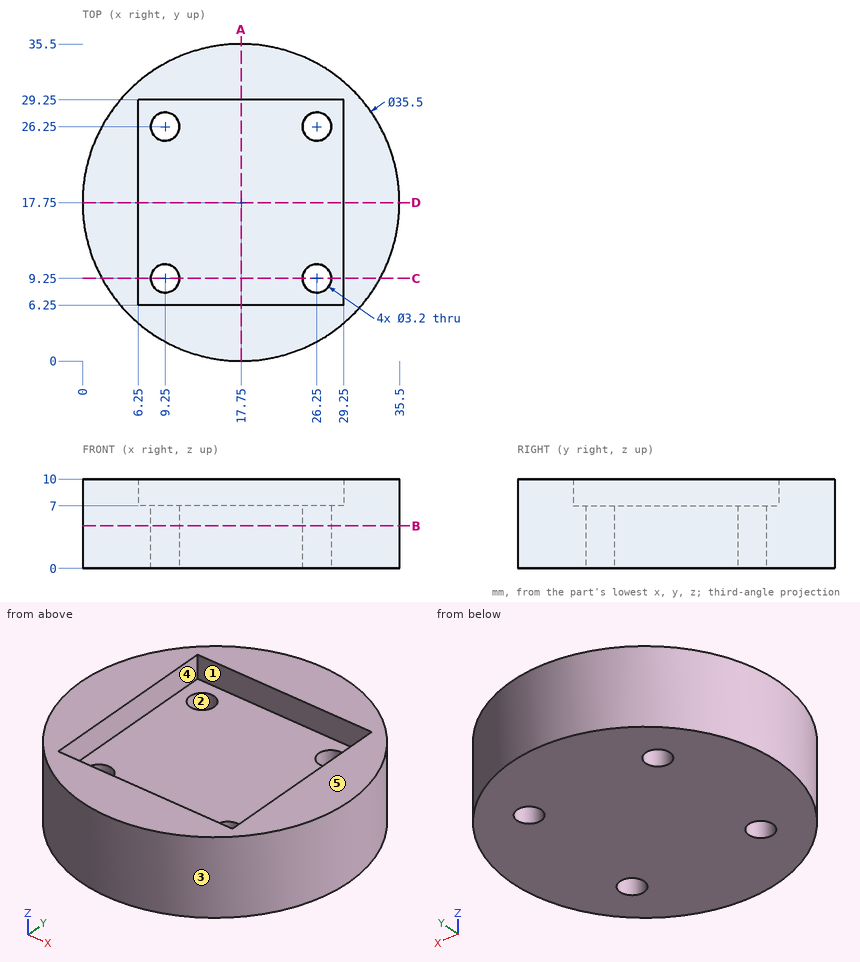
Here's the drawing with two shaded views (mm, measured from the low corner). I have some questions. A direction names the side the tool comes from. Give positions to 0.01 mm unless a question says otherwise; leave off trailing zeros. Order: outer loops, then holes, each group sorted by start corner. A loop starts at its lowest first (then second) coordinate and runs counter-clockwise, first axis right, second up. Notation, with made-up numbers: (-17, 2.25) -> (-4, 2.25) arc R32 cw to (-4, 35.25) -> close; hole circle Ø1 at (40, 17). An arc over 180 degrees is marked (long way). Use a Markdown table: item, result. Add a question column.
Item 1: I need wall thicknesses on line 1 (Y direction, x = 9.25, z = 5.25); line 2 (Y direction, x = 18, z = 8.25). Which ranges of each line are inside material? Lowest first, please.
Item 2: Will these pins go through, and if not, where does the flat tip stop? pin 1 (2.5 mm diameter, centred on x = 20, z = 8, fed in from +Y); pin 2 (2 mm diameter, centred on x = 25.5, z = 5.5, fed in from -Y); pin 3 (1.5 mm diameter, centred on y = 21.5, z = 9, fed in from +X).
Item 3: For the marked faces 1 and 2, which set-ups out of +Z, -Z, +X, -X, +Y, -Y let a thin tool reach every point of the face, with its end or its side?
Item 4: Imagine slicing it at A-A on x = 17.75. Please give me the cut outline in (y, z).
Item 5: Imagine slicing it at B-B on z = 4.75. Please give me the cut outline in (x, y), plus the area to 3 significant figures.
Item 6: Imagine slicing it at C-C on y = 9.25. Please give me the cut outline in (x, z).
Item 7: If we mould it in two halves opening along X, with no side actions, what happens to the marked faces 3, 4 and 5? For each: pulls with the +X half, pulls with the -X half, needs draft (parallel to the pull), parting line crosses it, or undercut.
Data:
| question | item | result |
|---|---|---|
| 1 | line 1 | y = 2.17 to 7.65, 10.85 to 24.65, 27.85 to 33.33 |
| 1 | line 2 | y = 0 to 6.25, 29.25 to 35.5 |
| 2 | pin 1 | stops at y = 35.47 |
| 2 | pin 2 | stops at y = 1.33 |
| 2 | pin 3 | stops at x = 35.24 |
| 3 | face 1 | +Z |
| 3 | face 2 | +Z, -Z |
| 4 | outline | (0, 0) -> (35.5, 0) -> (35.5, 10) -> (29.25, 10) -> (29.25, 7) -> (6.25, 7) -> (6.25, 10) -> (0, 10) -> close |
| 5 | outline | circle Ø35.5 at (17.75, 17.75); hole circle Ø3.2 at (9.25, 9.25); hole circle Ø3.2 at (9.25, 26.25); hole circle Ø3.2 at (26.25, 9.25); hole circle Ø3.2 at (26.25, 26.25) |
| 5 | area | 958 mm² |
| 6 | outline | (2.17, 0) -> (7.65, 0) -> (7.65, 7) -> (6.25, 7) -> (6.25, 10) -> (2.17, 10) -> close; (10.85, 0) -> (24.65, 0) -> (24.65, 7) -> (10.85, 7) -> close; (27.85, 0) -> (33.33, 0) -> (33.33, 10) -> (29.25, 10) -> (29.25, 7) -> (27.85, 7) -> close |
| 7 | face 3 | parting line crosses it |
| 7 | face 4 | undercut |
| 7 | face 5 | needs draft |
